from build123d import *

# Parameters (mm, degrees)
BOSS_EXTRUDE1_DEPTH = 76.2
SKETCH3_R           = 4.0005
BOSS_EXTRUDE2_DEPTH = 6.35
SKETCH4_W           = 19.05
SKETCH4_H           = 25.4
SKETCH4_R           = 3.175
BOSS_EXTRUDE3_DEPTH = 6.35
FILLET1_R           = 6.35


with BuildPart() as part:
    # Sketch2 → Boss-Extrude1 (new body)
    with BuildSketch(Plane(origin=(0, 0, 0), x_dir=(1, 0, 0), z_dir=(0, 1, 0))):
        Polygon((0, 22.225), (0, 0), (25.4, 0), (25.4, 22.225), (19.05, 22.225), (19.05, 6.35), (6.35, 6.35), (6.35, 22.225), align=None)
    extrude(amount=BOSS_EXTRUDE1_DEPTH)

    # Sketch3 → Boss-Extrude2 (add)
    with BuildSketch(Plane.XY):
        with BuildLine():
            Line((12.7, 50.8), (-25.4, 50.8))
            ThreePointArc((-25.4, 50.8), (-38.1, 38.1), (-25.4, 25.4))
            Line((-25.4, 25.4), (12.7, 25.4))
            ThreePointArc((12.7, 25.4), (25.4, 38.1), (12.7, 50.8))
        make_face()
        with Locations((-25.4, 38.1)):
            Circle(SKETCH3_R, mode=Mode.SUBTRACT)
    extrude(amount=-BOSS_EXTRUDE2_DEPTH)

    # Sketch4 → Boss-Extrude3 (add)
    # profile 1 of 2: a face of its own
    with BuildSketch(Plane(origin=(0, 0, -22.225), x_dir=(-1, 0, 0), z_dir=(0, 0, -1))):
        with Locations((-34.925, 38.1)):
            Rectangle(SKETCH4_W, SKETCH4_H)
        with Locations((-34.925, 38.1)):
            Circle(SKETCH4_R, mode=Mode.SUBTRACT)
    # profile 2 of 2: a face of its own
    with BuildSketch(Plane(origin=(0, 0, -22.225), x_dir=(-1, 0, 0), z_dir=(0, 0, -1))):
        with Locations((9.525, 38.1)):
            Rectangle(SKETCH4_W, SKETCH4_H)
        with Locations(Location((9.525, 38.1, 0), (0, 0, 180))):
            Circle(SKETCH4_R, mode=Mode.SUBTRACT)
    extrude(amount=-BOSS_EXTRUDE3_DEPTH)

    # Fillet1
    fillet1_edges = [part.edges().sort_by_distance(p)[0] for p in [
        (44.45, 25.4, -19.05),
        (44.45, 50.8, -19.05),
        (-19.05, 50.8, -19.05),
        (-19.05, 25.4, -19.05),
    ]]
    fillet(fillet1_edges, radius=FILLET1_R)


solid = part.part
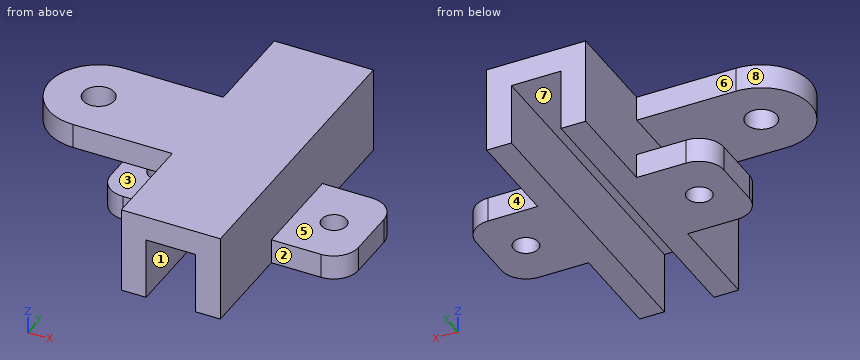
The listing builds one solid part. Answer for the finished solid, in the listing's coordinates (mm). Face numbers are marked on the shaded views. A direction names the side the tool comes from. Coordinates: 2 decimals unless noted, no trailing zeros. Loops run counter-clockwise (first coordinate to the right, second up) from the corner with the lowest first, then second, coordinate; pieces in that order, holes last. Notation, with made-up numbers: (-11.5, -37) -> (2.5, -37) arc R23 ccw to (2.5, -22) -> close; hole circle Ø3 at (26, -28). An arc over 180 degrees is marked (long way). Write item = value, one per line. Start each with the question number.
1) A cutting plane is placed at A-A (z = -18.5). Give the vertices of the cut face in (x, y) (3 decimals).
2) A cutting plane is placed at B-B (y = 38.1). Count the separate pieces of the cut face and the enclosed holes in it, then the cut area to 3 significant figures.
3) A cutting plane is placed at D-D (y = 12). Give the vertices of the cut face in (x, z) (3 decimals).
4) Given pin 1 Ø1.9 at (x, z) = (-8.5, -17.5) entering from -Y; pin 2 Ø5 at (y, z) = (16.5, -18.5) entering from +X; pin 3 Ø7 at (x, z) = (32.5, -20.5) entering from +Y; pin 4 Ø7 at (x, y) = (-25.4, 38.1) entering from +Z, each flat-ended and moving along its own axis, determine where each tip first touches the part or whether it passes through.
5) A cutting plane is placed at C-C (z = -14). Give the vertices of the cut face in (x, y), then the cut area to 3 significant figures.
6) The mould has two halves that part along X. Classify the marked faces 6, 7 and 8: released by +X, released by -X, zero draft, split by the parting line, or undercut.
7) Straight lines are drawn through the part: line 1 (Y direction, x = -25.4, z = -3.75); line 2 (X direction, y = 6, z = -16.5); line 3 (Z direction, x = -2, y = 47) (3 decimals). For each, find the intervals that lie inside material, in ascending order. Write a range as from..to.
8) A tool of negligible diameter and unlimited length cuts with its end or side. For the marked faces 1, 2, 3, 4 and 5, from which of +Z, -Z, +X, -X, +Y, -Y can it reach the whole face along a straight path? Write none if from no direction.
Responses:
q1.outline = (-19.05, 31.75) arc R6.35 ccw to (-12.7, 25.4) -> (0, 25.4) -> (0, 0) -> (6.35, 0) -> (6.35, 76.2) -> (0, 76.2) -> (0, 50.8) -> (-12.7, 50.8) arc R6.35 ccw to (-19.05, 44.45) -> close; (19.05, 0) -> (25.4, 0) -> (25.4, 25.4) -> (38.1, 25.4) arc R6.35 ccw to (44.45, 31.75) -> (44.45, 44.45) arc R6.35 ccw to (38.1, 50.8) -> (25.4, 50.8) -> (25.4, 76.2) -> (19.05, 76.2) -> close; hole circle Ø6.35 at (-9.525, 38.1); hole circle Ø6.35 at (34.925, 38.1)
q2.separate_pieces = 4
q2.enclosed_holes = 0
q2.area = 715 mm²
q3.outline = (0, -22.225) -> (6.35, -22.225) -> (6.35, -6.35) -> (19.05, -6.35) -> (19.05, -22.225) -> (25.4, -22.225) -> (25.4, 0) -> (0, 0) -> close
q4.pin_1 = 25.4
q4.pin_2 = 25.4
q4.pin_3 = 50.8
q4.pin_4 = through
q5.outline = (0, 0) -> (6.35, 0) -> (6.35, 76.2) -> (0, 76.2) -> close; (19.05, 0) -> (25.4, 0) -> (25.4, 76.2) -> (19.05, 76.2) -> close
q5.area = 968 mm²
q6.face_6 = zero draft
q6.face_7 = undercut
q6.face_8 = released by -X
q7.line_1 = 25.4..34.1, 42.1..50.8
q7.line_2 = 0..6.35, 19.05..25.4
q7.line_3 = -22.225..-15.875, -6.35..0
q8.face_1 = -Z, +Y, -Y
q8.face_2 = +Z, -Z, +X, -Y
q8.face_3 = -X, +Y, -Y
q8.face_4 = +Z, -Z, +X, +Y
q8.face_5 = +Z, +X, +Y, -Y
